Geometry check sheet. Reference: drawing and pictorial views, mm from the part's lowest x, y, z. Give positions to 0.01 mm unless a question says otherwise; leave off trailing zeros. Loops run counter-clockwise (first coordinate to the right, second up) from the corner with the lowest first, then second, coordinate; pieces in that order, holes last. Notation, with made-up numbers: (20, 35) - (68, 35) arc R27 ccw to (68, 64) - close; hole circle Ø4 at (39.25, 34.5). An arc over 180 degrees is marked (long way). Answer in a Markdown table with one row per item. Add a question column.
(1) Sectioned sample at A-A on x = 1171. Enter the section's corners in (y, z).
(2) Thickness scan on L1, parallel to X at y = 14.25, z = 250; L2, parallel to Z at x = 402, y = 5.25. Record the ranges inside material, lowest first.
(3) Sectioned sample at B-B on z = 326.5. Enter the section's corners in (x, y).
(4) Sectioned sample at C-C on y = 10.75. Enter the section's corners in (x, z).
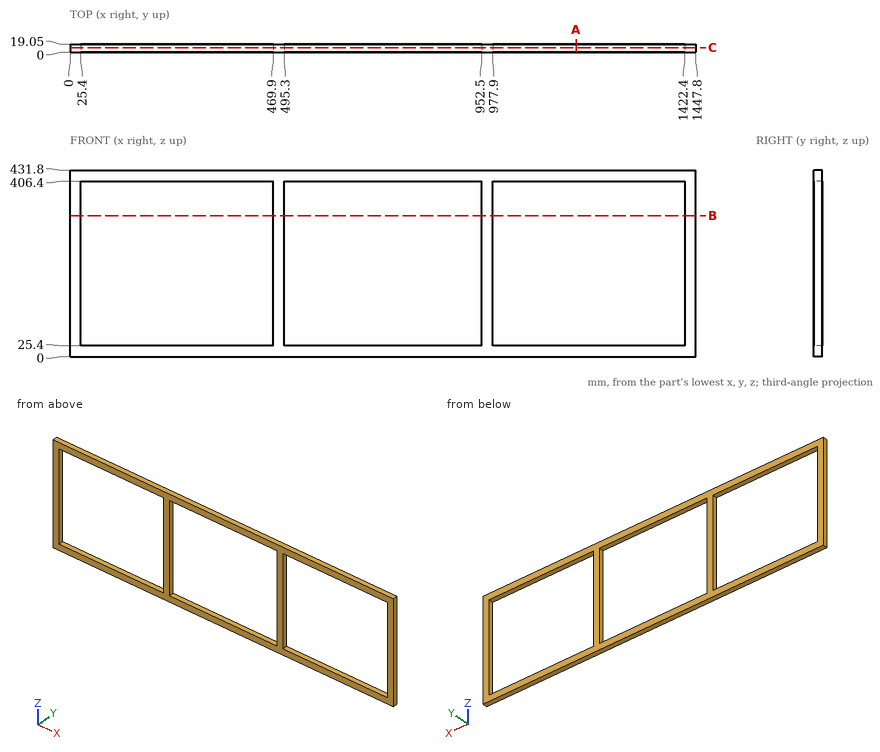
Reply:
| question | item | result |
|---|---|---|
| 1 | outline | (0, 0) - (19.05, 0) - (19.05, 25.4) - (0, 25.4) - close; (0, 406.4) - (19.05, 406.4) - (19.05, 431.8) - (0, 431.8) - close |
| 2 | L1 | 0 to 25.4, 469.9 to 495.3, 952.5 to 977.9, 1422.4 to 1447.8 |
| 2 | L2 | 0 to 25.4, 406.4 to 431.8 |
| 3 | outline | (0, 0) - (25.4, 0) - (25.4, 19.05) - (0, 19.05) - close; (469.9, 0) - (495.3, 0) - (495.3, 19.05) - (469.9, 19.05) - close; (952.5, 0) - (977.9, 0) - (977.9, 19.05) - (952.5, 19.05) - close; (1422.4, 0) - (1447.8, 0) - (1447.8, 19.05) - (1422.4, 19.05) - close |
| 4 | outline | (0, 0) - (1447.8, 0) - (1447.8, 431.8) - (0, 431.8) - close; hole (25.4, 25.4) - (469.9, 25.4) - (469.9, 406.4) - (25.4, 406.4) - close; hole (495.3, 25.4) - (952.5, 25.4) - (952.5, 406.4) - (495.3, 406.4) - close; hole (977.9, 25.4) - (1422.4, 25.4) - (1422.4, 406.4) - (977.9, 406.4) - close |
